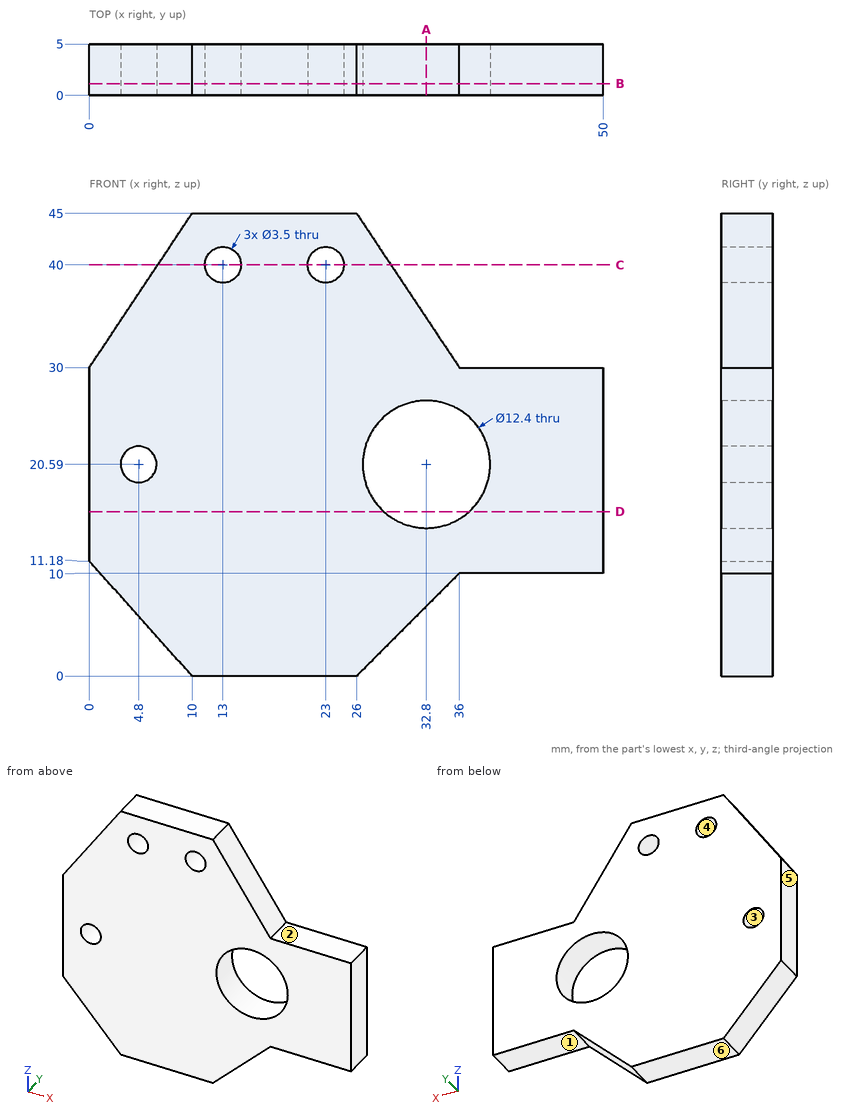
Study the drawing (mm; zero at the part's minimum x, y, z) and answer. A direction names the side the tool comes from. Give positions to 0.01 mm unless a question says otherwise; leave off trailing zeros. Write each loop counter-clockwise with the first axis right and the second up, starting at its lowest first coordinate (ties: lowest second). Pieces come first, ordered by that corner, then holes. Notation, with made-up numbers: (-0.5, 34.5) - (43.5, 34.5) arc R28 cw to (43.5, 72.5) - close; hole circle Ø4 at (9.25, 88.25). An arc over 180 degrees is marked (long way). One line per question, with ' | ' between items. Start each with the question number.
1. Given P1, Ø3, axis at x = 23, z = 40, coming from the -Y side, flat-ended and moving along its own axis, determine where the tip first touches the part or whether it passes through.
2. Section A-A, the plane x = 32.8 is taken. Determine the outline of the cut face in (y, z).
3. Determine the mould class of the marked faces 4, 5 and 6 for opening direction X: +X half, -X half, draft (parallel to the pull), parting line (faces both ways), or undercut.
4. Section B-B, the plane y = 1.15 is taken. Determine the outline of the cut face in (x, z).
5. For the marked faces 1, 2 and 3, determine the directions among +Z, -Z, +X, -X, +Y, -Y from which every point of the face is accessible in a straight line to the end or side of a thin tool.
6. Section D-D, the plane z = 16 is taken. Determine the outline of the cut face in (x, y), then the cut area to 3 significant figures.
7. Straight lines are drawn through the part: line 1 (X direction, y = 3.3, z = 21.5) (1 decimal); line 2 (X direction, y = 4.75, z = 39) (1 decimal); line 3 (Z direction, x = 45, y = 0.3). For each, find the intervals that lie inside material, in ascending order.
8. Section C-C, the plane z = 40 is taken. Determine the outline of the cut face in (x, y).
Result:
1) P1: passes through
2) outline: (0, 6.8) - (5, 6.8) - (5, 14.39) - (0, 14.39) - close; (0, 26.79) - (5, 26.79) - (5, 34.8) - (0, 34.8) - close
3) face 4: undercut | face 5: -X half | face 6: draft
4) outline: (0, 11.18) - (10, 0) - (26, 0) - (36, 10) - (50, 10) - (50, 30) - (36, 30) - (26, 45) - (10, 45) - (0, 30) - close; hole circle Ø3.5 at (4.8, 20.59); hole circle Ø3.5 at (13, 40); hole circle Ø3.5 at (23, 40); hole circle Ø12.4 at (32.8, 20.59)
5) face 1: -Z, +X, +Y, -Y | face 2: +Z, +X, +Y, -Y | face 3: +Y, -Y
6) outline: (0, 0) - (28.63, 0) - (28.63, 5) - (0, 5) - close; (36.97, 0) - (50, 0) - (50, 5) - (36.97, 5) - close | area: 208 mm2
7) line 1: x = 0 to 3.3, 6.3 to 26.7, 38.9 to 50 | line 2: x = 6 to 11.6, 14.4 to 21.6, 24.4 to 30 | line 3: z = 10 to 30
8) outline: (6.67, 0) - (11.25, 0) - (11.25, 5) - (6.67, 5) - close; (14.75, 0) - (21.25, 0) - (21.25, 5) - (14.75, 5) - close; (24.75, 0) - (29.33, 0) - (29.33, 5) - (24.75, 5) - close
